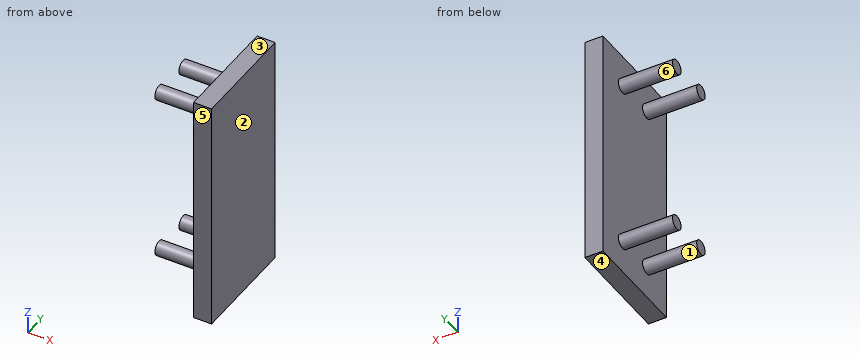
from build123d import *

# Parameters (mm, degrees)
SKETCH3_W           = 30
SKETCH3_H           = 65
BOSS_EXTRUDE1_DEPTH = 5
SKETCH4_R           = 2
BOSS_EXTRUDE2_DEPTH = 15


with BuildPart() as part:
    # Sketch3 → Boss-Extrude1 (new body)
    with BuildSketch(Plane.YZ):
        Rectangle(SKETCH3_W, SKETCH3_H)
    extrude(amount=BOSS_EXTRUDE1_DEPTH)

    # Sketch4 → Boss-Extrude2 (add)
    with BuildSketch(Plane(origin=(0, 0, 0), x_dir=(0, -1, 0), z_dir=(-1, 0, 0))):
        with Locations(Location((-5.7, -23.5, 0), (0, 0, 270))):
            Circle(SKETCH4_R)
        with Locations(Location((-5.7, 23.5, 0), (0, 0, 270))):
            Circle(SKETCH4_R)
        with Locations(Location((5.7, -23.5, 0), (0, 0, 270))):
            Circle(SKETCH4_R)
        with Locations(Location((5.7, 23.5, 0), (0, 0, 270))):
            Circle(SKETCH4_R)
    extrude(amount=BOSS_EXTRUDE2_DEPTH)


solid = part.part
For this review, take the finished solid that the model builds, in its own axes (mm). Face numbers are marked on the shaded views. A direction names the side the tool comes from. Coordinates: 2 decimals unless noted, no trailing zeros. Loops run counter-clockwise (first coordinate to the right, second up) from the corner with the lowest first, then second, coordinate; pieces in that order, holes last. Notation, with made-up numbers: (31.5, -20) - (70.5, -20) arc R26 cw to (70.5, 10) - close; hole circle Ø5 at (1, 16). An arc over 180 degrees is marked (long way). Return JSON: item names as keys, results as strings.
Item 1: Take a section at B-B (y = 4.5). Give the boundary of the cut face in (x, z).
Determined:
{"outline": "(-15, -25.1) - (0, -25.1) - (0, -32.5) - (5, -32.5) - (5, 32.5) - (0, 32.5) - (0, 25.1) - (-15, 25.1) - (-15, 21.9) - (0, 21.9) - (0, -21.9) - (-15, -21.9) - close"}
Item 2: Take a section at C-C (x = -6.25). Give the boundary of the cut face in (y, z).
Determined:
{"outline": "circle Ø4 at (-5.7, -23.5); circle Ø4 at (-5.7, 23.5); circle Ø4 at (5.7, -23.5); circle Ø4 at (5.7, 23.5)"}
Item 3: For the marked faces 1 and 2, list the 3-axis set-ups (+Z, -Z, +X, -X, +Y, -Y) from which the entire face can be reached by the end or side of a thin tool; tool diameter is ignored.
Determined:
{"face 1": "-X", "face 2": "+Z, -Z, +X, +Y, -Y"}
Item 4: For line 1 (X direction, y = 12.5, z = 0); line 2 (Z direction, x = -0.75, y = 6); line 3 (Y direction, x = -7.75, z = 22.5), list the stretches that pass through material, from the lowest coordinate up.
Determined:
{"line 1": "x = 0 to 5", "line 2": "z = -25.48 to -21.52, 21.52 to 25.48", "line 3": "y = -7.43 to -3.97, 3.97 to 7.43"}
Item 5: Insertion check: pin 1 (6 mm diameter, centred on x = -7, y = 7.5, fed in from +Z). The pin has a flat end and moves straight along its axis. Give the tip position at first contact, or say it passes through.
Determined:
{"pin 1": "stops at z = 25.5"}
Item 6: Mouldability with a two-part tool opening along Z and no side actions: class the marked faces 3, 4, 5 and 6 as pulls with the +Z half, pulls with the -Z half, needs draft (parallel to the pull), parting line crosses it, or undercut.
Determined:
{"face 3": "pulls with the +Z half", "face 4": "pulls with the -Z half", "face 5": "needs draft", "face 6": "undercut"}
Item 7: Take a section at A-A (z = -23.5). Give the boundary of the cut face in (x, y), then the cut area to 3 significant figures.
Determined:
{"outline": "(-15, -7.7) - (0, -7.7) - (0, -15) - (5, -15) - (5, 15) - (0, 15) - (0, 7.7) - (-15, 7.7) - (-15, 3.7) - (0, 3.7) - (0, -3.7) - (-15, -3.7) - close", "area": "270 mm2"}
Item 8: Take a section at D-D (y = -0.75). Give the boundary of the cut face in (x, z), then the cut area to 3 significant figures.
Determined:
{"outline": "(0, -32.5) - (5, -32.5) - (5, 32.5) - (0, 32.5) - close", "area": "325 mm2"}
